Check sheet for the modelled part. Datum: model origin and axes. Units: mm. A direction names the side the tool comes from. Round coordinates to 2 decimals unless told otherwise and drop trailing zeros. Order: outer loops, then holes, each group sorted by start corner. A loop starts at its lowest first (then second) coordinate and runs counter-clockwise, first axis right, second up.
Q1. Cross-section at D-D on x = -2.5. Record the cut outline in (y, z), then the cut area to 3 significant figures.
Q2. Scan lines: probe 1 along X at (y, z) = (-2.5, 0); probe 2 along Z at (x, y) = (0, 0.2). Record each from-to range of solid material in increasing order.
Q3. Cross-section at C-C on y = -0.55. Record the cut outline in (x, z), then the cut area to 3 significant figures.
Q4. Depth check by flat-ended pin: P1, Ø1, axis at x = 2, z = -1.5, coming from the -Y side; P2, Ø2, axis at x = 1.5, y = -2, coming from the +Z side; P3, Ø2, axis at y = -0.5, z = -1, coming from the +X side; P4, Ø1.5, axis at y = -2.5, z = -2.5, coming from the +X side. Enter the tip coordinate at first touch or a pass-through.
Q5. Cross-section at A-A on z = 0. Record the cut outline in (x, y).
Q6. Set-up check for faces 1 (the cylindrical face through (-3.746, 0.37, -0.165)), 2 (the flat face through (2, 0, 2)): record each of +Z, -Z, +X, -X, +Y, -Y from which the full face is reachable in a straight line by a thin tool's end or side.
Q7. Cross-section at B-B on x = 0. Record the cut outline in (y, z), then the cut area to 3 significant figures.
from build123d import *

# Parameters (mm, degrees)
SKETCH1_R           = 3.75
SKETCH1_R_2         = 1.5
BOSS_EXTRUDE1_DEPTH = 0.75
SKETCH2_R           = 2.25
SKETCH2_R_2         = 1.5
BOSS_EXTRUDE2_DEPTH = 5


with BuildPart() as part:
    # Sketch1 → Boss-Extrude1 (new body)
    with BuildSketch(Plane(origin=(0, 0, 0), x_dir=(1, 0, 0), z_dir=(0, 1, 0))):
        Circle(SKETCH1_R)
        Circle(SKETCH1_R_2, mode=Mode.SUBTRACT)
    extrude(amount=BOSS_EXTRUDE1_DEPTH)

    # Sketch2 → Boss-Extrude2 (add)
    with BuildSketch(Plane(origin=(0, 0.75, 0), x_dir=(1, 0, 0), z_dir=(0, 1, 0))):
        Circle(SKETCH2_R)
        Circle(SKETCH2_R_2, mode=Mode.SUBTRACT)
    extrude(amount=-BOSS_EXTRUDE2_DEPTH)


solid = part.part
Results found:
1. outline: (0, -2.8) - (0.75, -2.8) - (0.75, 2.8) - (0, 2.8) - close
1. area: 4.19 mm2
2. probe 1: x = -2.25 to -1.5, 1.5 to 2.25
2. probe 2: z = -3.75 to -1.5, 1.5 to 3.75
3. outline: circle Ø4.5 at (0, 0); hole circle Ø3 at (0, 0)
3. area: 8.84 mm2
4. P1: stops at y = -4.25
4. P2: stops at z = 2.19
4. P3: stops at x = 3.75
4. P4: stops at x = 1.41
5. outline: (-3.75, 0) - (-2.25, 0) - (-2.25, -4.25) - (-1.5, -4.25) - (-1.5, 0.75) - (-3.75, 0.75) - close; (1.5, -4.25) - (2.25, -4.25) - (2.25, 0) - (3.75, 0) - (3.75, 0.75) - (1.5, 0.75) - close
6. face 1: +Y, -Y
6. face 2: -Y
7. outline: (-4.25, -2.25) - (0, -2.25) - (0, -3.75) - (0.75, -3.75) - (0.75, -1.5) - (-4.25, -1.5) - close; (-4.25, 1.5) - (0.75, 1.5) - (0.75, 3.75) - (0, 3.75) - (0, 2.25) - (-4.25, 2.25) - close
7. area: 9.75 mm2
